Part model, mm, in its own coordinate system. Face numbers are marked on the shaded views. A direction names the side the tool comes from. Round coordinates to 2 decimals unless told otherwise and drop trailing zeros.
1) Drop flat-ended pins along their axis: P1, Ø3.5, axis at x = -12.5, y = 5, coming from the -Z side; P2, Ø1.5, axis at x = 15, y = 3.5, coming from the +Z side; P3, Ø6, axis at y = 7.5, z = 59.5, coming from the +X side. Give the stop position or say it passes through.
2) Band-saw the part on A-A, the plane y = 5. State how many separate pieces and enclosed holes the cut face has, then the cut area to 3 significant figures.
3) 3-axis set-ups, long thin cutter, end or side, ignore diameter. For the marked faces 4 and 5: which of +Z, -Z, +X, -X, +Y, -Y reach the whole face in a straight line?
4) Probe line 1 (Y direction, x = 12.5, z = 56); line 2 (X direction, y = 2, z = 64.75); line 3 (Y direction, x = 12.5, z = 69.25). List the from-to ranges inside material, lowest first.
5) Mould opens along X. For the marked faces 1, 2 and 3 say: +X half, -X half, draft (parallel to the pull), parting line (faces both ways), or undercut.
from build123d import *

# Parameters (mm, degrees)
BOSS_EXTRUDE1_DEPTH = 10
FILLET1_R           = 5
SKETCH2_R           = 1.5
CUT_EXTRUDE1_DEPTH  = 36.878807745
CUT_EXTRUDE2_START  = -10
SKETCH2_3_R         = 4
SKETCH2_3_R_2       = 1.5
CUT_EXTRUDE2_DEPTH  = 26.878807842
CHAMFER1_SIZE       = 0.381


with BuildPart() as part:
    # Sketch1 → Boss-Extrude1 (new body)
    with BuildSketch(Plane(origin=(0, 0, 0), x_dir=(1, 0, 0), z_dir=(0, 1, 0))):
        with BuildLine():
            Line((-6.330284354, -50.5), (-24.9949995, -50.5))
            ThreePointArc((-24.9949995, -50.5), (0, -75), (24.9949995, -50.5))
            Line((24.9949995, -50.5), (6.330284354, -50.5))
            ThreePointArc((6.330284354, -50.5), (0, -56.35), (-6.330284354, -50.5))
        make_face()
    extrude(amount=BOSS_EXTRUDE1_DEPTH)

    # Fillet1
    fillet1_edges = [part.edges().sort_by_distance(p)[0] for p in [
        (24.9949995, 5, 50.5),
        (-24.9949995, 5, 50.5),
    ]]
    fillet(fillet1_edges, radius=FILLET1_R)

    # Sketch2 → Cut-Extrude1 (cut, through all)
    with BuildSketch(Plane(origin=(0, 0, 50.5), x_dir=(-1, 0, 0), z_dir=(0, 0, -1))):
        with Locations((-12.5, 5)):
            Circle(SKETCH2_R)
        with Locations((12.5, 5)):
            Circle(SKETCH2_R)
    extrude(amount=-CUT_EXTRUDE1_DEPTH, mode=Mode.SUBTRACT)

    # Sketch2<3> → Cut-Extrude2 (cut, through all)
    # profile 1 of 2: a face of its own
    with BuildSketch(Plane(origin=(0, 0, 50.5), x_dir=(-1, 0, 0), z_dir=(0, 0, -1)).offset(CUT_EXTRUDE2_START)):
        with Locations((-12.5, 5)):
            Circle(SKETCH2_3_R)
        with Locations((-12.5, 5)):
            Circle(SKETCH2_3_R_2, mode=Mode.SUBTRACT)
    # profile 2 of 2: a face of its own
    with BuildSketch(Plane(origin=(0, 0, 50.5), x_dir=(-1, 0, 0), z_dir=(0, 0, -1)).offset(CUT_EXTRUDE2_START)):
        with Locations((12.5, 5)):
            Circle(SKETCH2_3_R)
        with Locations((12.5, 5)):
            Circle(SKETCH2_3_R_2, mode=Mode.SUBTRACT)
    extrude(amount=-CUT_EXTRUDE2_DEPTH, mode=Mode.SUBTRACT)

    # Chamfer1
    chamfer1_edges = [part.edges().sort_by_distance(p)[0] for p in [
        (0, 0, 75),
        (12.779584438, 10, 50.5),
        (0, 10, 75),
        (-12.779584438, 0, 50.5),
        (23.221064379, 0, 52.489601355),
        (0, 10, 56.35),
        (-23.221064379, 0, 52.489601355),
        (-12.779584438, 10, 50.5),
        (23.221064379, 10, 52.489601355),
        (-23.221064379, 10, 52.489601355),
        (14, 5, 50.5),
        (-11, 5, 50.5),
        (14, 5, 60.5),
        (-11, 5, 60.5),
        (0, 0, 56.35),
        (12.779584438, 0, 50.5),
    ]]
    chamfer(chamfer1_edges, length=CHAMFER1_SIZE)


solid = part.part
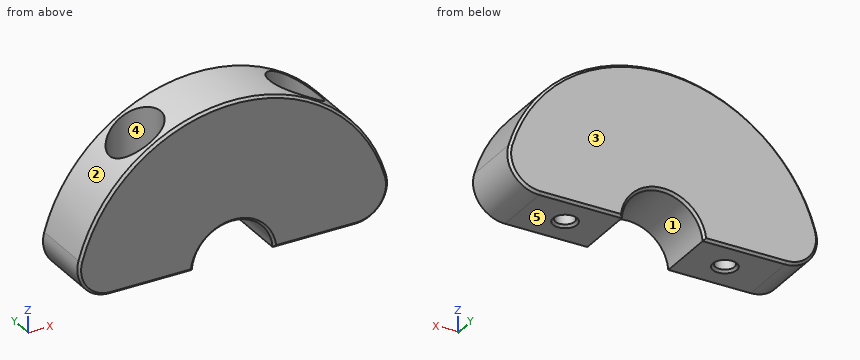
Reported:
1. P1: stops at z = 50.63
1. P2: stops at z = 60.5
1. P3: stops at x = 24.13
2. separate pieces: 3
2. enclosed holes: 0
2. area: 647 mm2
3. face 4: +Z
3. face 5: -Z, +X, -X, +Y, -Y
4. line 1: y = 0 to 3.5, 6.5 to 10
4. line 2: x = -20.19 to -15.15, -9.85 to 9.85, 15.15 to 20.19
4. line 3: y = 0 to 1, 9 to 10
5. face 1: undercut
5. face 2: parting line
5. face 3: draft
